```python
from build123d import *

# Parameters (mm, degrees)
SKETCH1_R           = 25.5
BOSS_EXTRUDE1_DEPTH = 1.5
SKETCH2_R           = 26
BOSS_EXTRUDE2_DEPTH = 1
SKETCH3_R           = 0.55
CUT_EXTRUDE1_DEPTH  = 37.783148315


with BuildPart() as part:
    # Sketch1 → Boss-Extrude1 (new body)
    with BuildSketch(Plane(origin=(0, 0, 0), x_dir=(1, 0, 0), z_dir=(0, 1, 0))):
        with Locations(Location((0, 0, 0), (0, 0, 270))):
            Circle(SKETCH1_R)
    extrude(amount=-BOSS_EXTRUDE1_DEPTH)

    # Sketch2 → Boss-Extrude2 (add)
    with BuildSketch(Plane(origin=(0, -1.5, 0), x_dir=(-1, 0, 0), z_dir=(0, -1, 0))):
        with Locations(Location((0, 0, 0), (0, 0, 90))):
            Circle(SKETCH2_R)
    extrude(amount=-BOSS_EXTRUDE2_DEPTH)

    # Sketch3 → Cut-Extrude1 (cut, through all)
    with BuildSketch(Plane(origin=(0, -0.5, 0), x_dir=(1, 0, 0), z_dir=(0, 1, 0))):
        with Locations(Location((0, 0, 0), (0, 0, 270))):
            Circle(SKETCH3_R)
    extrude(amount=-CUT_EXTRUDE1_DEPTH, mode=Mode.SUBTRACT)

    # Sketch4 → Cut-Revolve1 (revolve, cut)
    with BuildSketch(Plane.XY, mode=Mode.PRIVATE) as cut_revolve1_sk:
        Polygon((-4.35, -1.5), (0, -1.5), (0, 0), (-0.55, 0), (-0.55, -0.2), align=None)
    revolve(cut_revolve1_sk.sketch.rotate(Axis((0, -1.5, 0), (0, 1, 0)), 270), axis=Axis((0, -1.5, 0), (0, 1, 0)), mode=Mode.SUBTRACT)


solid = part.part
```
Could you check a few things on this model? Use its own coordinates, in mm. A direction names the side the tool comes from. Coordinates: 2 decimals unless noted, no trailing zeros. Loops run counter-clockwise (first coordinate to the right, second up) from the corner with the lowest first, then second, coordinate; pieces in that order, holes last.
1) Which directions (+Z, -Z, +X, -X, +Y, -Y) give clear straight access to the entire face, cutting with the end or side of a thin tool? Please do faces 1 (the face through (-17.2, -0.5, -19.1)), 2 (the face through (0, -1.5, -5)).
Reported:
face 1: +Y
face 2: +Z, -Z, +X, -X, -Y
2) Imagine slicing it at B-B (z = 15.5). List the corners of the cut face in (x, y) for me.
Reported:
outline: (-20.87, -1.5) - (20.87, -1.5) - (20.87, -0.5) - (20.25, -0.5) - (20.25, 0) - (-20.25, 0) - (-20.25, -0.5) - (-20.87, -0.5) - close
3) Imagine slicing it at A-A (x = -6). List the corners of the cut face in (y, z) for me, and give its area (3 significant figures).
Reported:
outline: (-1.5, -25.3) - (-0.5, -25.3) - (-0.5, -24.78) - (0, -24.78) - (0, 24.78) - (-0.5, 24.78) - (-0.5, 25.3) - (-1.5, 25.3) - close
area: 75.4 mm2
4) Thinking about a two-plate mould opening in Z: for faces 3 (the face through (0.77, -0.28, 0.17)), 4 (the face through (-15.821, -1.007, 20.633)), 5 (the face through (-5, 0, 0)), which applies, released by +Z, released by -Z, zero draft, split by the parting line, or undercut?
Reported:
face 3: undercut
face 4: split by the parting line
face 5: zero draft
5) Will this pin go through, and if not, where does the flat tip stop? pin 1 Ø0.9 at (x, z) = (0, 0) entering from -Y.
Reported:
pin 1: passes through
6) Please list where these lines run through material, in increasing order: line 1 along X through (y, z) = (-0.05, 0); line 2 along Z through (x, y) = (-18, -0.4); line 3 along X through (y, z) = (-0.85, 12.5).
Reported:
line 1: x = -25.5 to -0.55, 0.55 to 25.5
line 2: z = -18.06 to 18.06
line 3: x = -22.8 to 22.8
